Here's how the part is built. I have some questions about the finished solid (model axes, mm). A direction names the side the tool comes from. Round coordinates to 2 decimals unless told otherwise and drop trailing zeros. Loops run counter-clockwise (first coordinate to the right, second up) from the corner with the lowest first, then second, coordinate; pieces in that order, holes last. Notation, with made-up numbers: M -32,84 L 9,84 A17 ccw 9,98 Z; hole C 39,-27.75 d8. An arc over 180 degrees is marked long. Write each question's results on one line, items separated by ' | '. Start each with the question number.
```python
from build123d import *

# Parameters (mm, degrees)
F9_R          = 2.5
F10_DEPTH     = 24.5
F11_DEPTH     = 6.75
F12_DEPTH     = 14
F13_T2_ANGLE  = 157.8095212227
F13_T6_DEPTH  = 3.4652909658
F13_S7_R      = 4.5
F13_T8_DEPTH  = 3
F13_T12_DEPTH = 3.4652909658
F13_S13_R     = 4.5
F13_T14_DEPTH = 3
F13_T16_ANGLE = 157.8095212227
F13_T20_DEPTH = 3.4652909658
F13_S21_R     = 4.5
F13_T22_DEPTH = 3
F13_T26_DEPTH = 3.4652909658
F13_S27_R     = 4.5
F13_T28_DEPTH = 3


# Not quite as in the source:
# - a fillet or chamfer that OpenCascade refuses, or shapes differently, is made with other operations: its cross-section is extruded or revolved along the edge and cut away or added


with BuildPart() as f7:
    # F6 (on Top) → F7 (revolve)
    with BuildSketch(Plane.XY):
        with BuildLine():
            Line((-4, 4.5), (-4, 2.5))
            Line((-4, 2.5), (4, 2.5))
            Line((4, 2.5), (4, 4.5))
            ThreePointArc((4, 4.5), (3.5461149614, 5.1104772433), (3, 5.6400549446))
            ThreePointArc((3, 5.6400549446), (0, 6.716990566), (-3, 5.6400549446))
            ThreePointArc((-3, 5.6400549446), (-3.5461149614, 5.1104772433), (-4, 4.5))
        make_face()
        with BuildLine():
            Line((-3, 7.1961524227), (-3, 5.6400549446))
            ThreePointArc((-3, 5.6400549446), (0, 6.716990566), (3, 5.6400549446))
            Line((3, 5.6400549446), (3, 7.1961524227))
            ThreePointArc((3, 7.1961524227), (0, 8), (-3, 7.1961524227))
        make_face()
    revolve(axis=Axis((0, 0, 0), (1, 0, 0)))

    # F9 (on offset) → F10 (join)
    with BuildSketch(Plane.XZ.offset(-27)):
        with BuildLine():
            ThreePointArc((-4.5, 0), (0, -4.5), (4.5, 0))
            ThreePointArc((4.5, 0), (0, 4.5), (-4.5, 0))
        make_face()
        Circle(F9_R, mode=Mode.SUBTRACT)
        Circle(F9_R)
    extrude(amount=F10_DEPTH)

    # F9 (on offset) → F11 (join)
    with BuildSketch(Plane.XZ.offset(-27)):
        with BuildLine():
            ThreePointArc((-4.5, 0), (0, 4.5), (4.5, 0))
            Line((4.5, 0), (4.5, 2.1794494718))
            ThreePointArc((4.5, 2.1794494718), (0, 5), (-4.5, 2.1794494718))
            Line((-4.5, 2.1794494718), (-4.5, 0))
        make_face()
        with BuildLine():
            Line((4.5, -2.1794494718), (4.5, 0))
            ThreePointArc((4.5, 0), (0, -4.5), (-4.5, 0))
            Line((-4.5, 0), (-4.5, -2.1794494718))
            ThreePointArc((-4.5, -2.1794494718), (0, -5), (4.5, -2.1794494718))
        make_face()
    extrude(amount=F11_DEPTH)

    # F9 (on offset) → F12 (cut)
    with BuildSketch(Plane.XZ.offset(-27)):
        Circle(F9_R)
    extrude(amount=F12_DEPTH, mode=Mode.SUBTRACT)

    # F13: chamfer of 0.5 on 6 edges, made by hand

    # F13_s1 → F13_t2 (revolve, cut)
    with BuildSketch(Plane(origin=(0, 0, 0), x_dir=(0, 1, 0), z_dir=(0.1924404319, 0, -0.9813086569))):
        Polygon((20.25, 4.5), (20.75, 5), (20.25, 5), align=None)
    revolve(axis=Axis((0, 20.25, 0), (0, -1, 0)), revolution_arc=F13_T2_ANGLE, mode=Mode.SUBTRACT)


with BuildPart() as f13_tool4:
    # F13_s5 → F13_t6 (new body)
    with BuildSketch(Plane.XY):
        Polygon((4, 20.25), (4.5, 20.75), (4.5, 20.25), align=None)
    extrude(amount=F13_T6_DEPTH)

    # F13_s7 → F13_t8 (cut, symmetric)
    with BuildSketch(Plane.XZ.offset(-20.5)):
        Circle(F13_S7_R)
    extrude(amount=F13_T8_DEPTH, both=True, mode=Mode.SUBTRACT)


with BuildPart() as f7_1:
    add(f7.part)

    # F13_t3: cut F13_tool4
    add(f13_tool4.part, mode=Mode.SUBTRACT)


with BuildPart() as f13_tool10:
    # F13_s11 → F13_t12 (new body)
    with BuildSketch(Plane.XY.offset(3.4652909658)):
        Polygon((-4, 20.25), (-4.5, 20.75), (-4.5, 20.25), align=None)
    extrude(amount=-F13_T12_DEPTH)

    # F13_s13 → F13_t14 (cut, symmetric)
    with BuildSketch(Plane.XZ.offset(-20.5)):
        Circle(F13_S13_R)
    extrude(amount=F13_T14_DEPTH, both=True, mode=Mode.SUBTRACT)


with BuildPart() as f7_2:
    add(f7_1.part)

    # F13_t9: cut F13_tool10
    add(f13_tool10.part, mode=Mode.SUBTRACT)

    # F13_s15 → F13_t16 (revolve, cut)
    with BuildSketch(Plane(origin=(0, 0, 0), x_dir=(0, 1, 0), z_dir=(-0.1924404319, 0, 0.9813086569))):
        Polygon((20.25, 4.5), (20.75, 5), (20.25, 5), align=None)
    revolve(axis=Axis((0, 20.25, 0), (0, -1, 0)), revolution_arc=F13_T16_ANGLE, mode=Mode.SUBTRACT)


with BuildPart() as f13_tool18:
    # F13_s19 → F13_t20 (new body)
    with BuildSketch(Plane.XY.offset(-3.4652909658)):
        Polygon((4, 20.25), (4.5, 20.75), (4.5, 20.25), align=None)
    extrude(amount=F13_T20_DEPTH)

    # F13_s21 → F13_t22 (cut, symmetric)
    with BuildSketch(Plane.XZ.offset(-20.5)):
        Circle(F13_S21_R)
    extrude(amount=F13_T22_DEPTH, both=True, mode=Mode.SUBTRACT)


with BuildPart() as f7_3:
    add(f7_2.part)

    # F13_t17: cut F13_tool18
    add(f13_tool18.part, mode=Mode.SUBTRACT)


with BuildPart() as f13_tool24:
    # F13_s25 → F13_t26 (new body)
    with BuildSketch(Plane.XY):
        Polygon((-4, 20.25), (-4.5, 20.75), (-4.5, 20.25), align=None)
    extrude(amount=-F13_T26_DEPTH)

    # F13_s27 → F13_t28 (cut, symmetric)
    with BuildSketch(Plane.XZ.offset(-20.5)):
        Circle(F13_S27_R)
    extrude(amount=F13_T28_DEPTH, both=True, mode=Mode.SUBTRACT)


with BuildPart() as f7_4:
    add(f7_3.part)

    # F13_t23: cut F13_tool24
    add(f13_tool24.part, mode=Mode.SUBTRACT)

    # F6 (on Top) → F14 (revolve, cut)
    with BuildSketch(Plane.XY):
        with BuildLine():
            Line((4, 4.5), (4, 2.5))
            Line((4, 2.5), (6, 2.5))
            Line((6, 2.5), (6, 15.4385846811))
            Line((6, 15.4385846811), (3, 7.1961524227))
            Line((3, 7.1961524227), (3, 5.6400549446))
            ThreePointArc((3, 5.6400549446), (3.5461149614, 5.1104772433), (4, 4.5))
        make_face()
        with BuildLine():
            Line((-6, 2.5), (-4, 2.5))
            Line((-4, 2.5), (-4, 4.5))
            ThreePointArc((-4, 4.5), (-3.5461149614, 5.1104772433), (-3, 5.6400549446))
            Line((-3, 5.6400549446), (-3, 7.1961524227))
            Line((-3, 7.1961524227), (-6, 15.4385846811))
            Line((-6, 15.4385846811), (-6, 2.5))
        make_face()
    revolve(axis=Axis((0, 0, 0), (1, 0, 0)), mode=Mode.SUBTRACT)


solid = f7_4.part
```
Item 1: If we section it at B-B on y = 23: Please give me the cut outline in (x, z), and give its area (3 significant figures).
Item 2: I'm going to push flat-ended pins straight in: pin 1 (2 mm diameter, centred on y = 3.5, z = 0.5, fed in from +X); pin 2 (1.3 mm diameter, centred on y = 6, z = 1.5, fed in from -X); pin 3 (1 mm diameter, centred on y = 3.5, z = 0.5, fed in from -X); pin 4 (4 mm diameter, centred on y = 0, z = 0, fed in from -X). Where does each tip first touch, or does it pass through?
Item 3: I need wall thicknesses on L1, parallel to Z at x = 0, y = 22.5; L2, parallel to X at y = 4.5, z = 4.5; L3, parallel to Z at x = 0, y = 19.5. Which ranges of each line are inside material? Lowest first, please.
Item 4: If we section it at A-A on y = 16: Please give me the cut outline in (x, z).
Item 5: Which directions (+Z, -Z, +X, -X, +Y, -Y) give clear straight access to the entire face, cutting with the end or side of a thin tool? Please do faces 5 (the face through (0, 24, 5)), 6 (the face through (-0.54, 20.1, -2.44)), 7 (the face through (-0.07, 20.39, -4.64)), 8 (the face through (0.06, -0.54, -2.44)).
Item 6: If we mould it in two halves opening along Z, with no side actions, what happens to faces 1 (the face through (0, 24, -5)), 2 (the face through (0, 13, 0)), 3 (the face through (0.07, 20.39, 4.64)), 4 (the face through (4.5, 24, 0))? For each: released by +Z, released by -Z, zero draft, split by the parting line, or undercut.
Numbers:
1) outline: M -4.5,-2.18 A5 ccw 4.5,-2.18 L 4.5,2.18 A5 ccw -4.5,2.18 Z; hole C 0,0 d5 | area: 56.0 mm²
2) pin 1: x = 4 | pin 2: x = -3.12 | pin 3: x = -4 | pin 4: through
3) L1: -5 to -2.5, 2.5 to 5 | L2: -3 to 3 | L3: -4.5 to -2.5, 2.5 to 4.5
4) outline: C 0,0 d9; hole C 0,0 d5
5) face 5: +Z, +Y | face 6: +Y | face 7: -Z | face 8: +X, -X
6) face 1: released by -Z | face 2: undercut | face 3: released by +Z | face 4: zero draft
